Autodesk Inventor part; units mm, degrees
ref_plane "YZ Plane" through (0, 0, 0) normal (1, 0, 0) x (0, 1, 0)
ref_plane "XZ Plane" through (0, 0, 0) normal (0, 1, 0) x (-1, 0, 0)
ref_plane "XY Plane" through (0, 0, 0) normal (0, 0, 1) x (1, 0, 0)
sketch "Sketch1" plane through (0, 0, 0) normal (0, 0, 1) x (1, 0, 0)
  line L0 (457.2, 0) -> (457.2, 19.05)
  line L1 (457.2, -133.35) -> (457.2, 0)
  line L2 (0, 0) -> (0, -133.35)
  line L3 (457.2, 19.05) -> (1981.2, -133.35)
  line L4 (1789.7499, -133.35) -> (457.2, -0.095)
  line L5 (1789.7499, -133.35) -> (1981.2, -133.35)
  dimension "d3" = 19.05
  dimension "d4" = 1981.2
extrude "Extrusion1" add sketch "Sketch1" against normal blind 457.2
properties part number "Ramp1"
Geometry check sheet. Reference: the model listing, model coordinates, mm. Give positions to 0.01 mm unless a question says otherwise; leave off trailing zeros. Write each loop counter-clockwise with the first axis right and the second up, starting at its lowest first coordinate (ties: lowest second). Pieces come first, ordered by that corner, then holes.
1) Section check B-B, the plane x = 1686. Record the boundary of the cut face in (y, z) (3 decimals).
2) Section check A-A, the plane z = -96. Record the boundary of the cut face in (x, y) (3 decimals).
3) Gauge pin test, flat ends, axial feed: pin 1 (6 mm diameter, centred on x = 1481, z = -392, fed in from -Y) (3 decimals); pin 2 (2 mm diameter, centred on x = 961, z = -233, fed in from -Y) (3 decimals); pin 3 (10 mm diameter, centred on x = 1115.5, z = -358.5, fed in from -Y) (3 decimals). Record the tip position at first contact, or that the pin passes through.
4) Material ranges on L1, parallel to Y at x = 1027.5, z = -341.5 (3 decimals); L2, parallel to Y at x = 1285, z = -310 (3 decimals), recorded low to high.
Computed:
1. outline: (-122.975, -457.2) - (-103.83, -457.2) - (-103.83, 0) - (-122.975, 0) - close
2. outline: (457.2, -0.095) - (1789.75, -133.35) - (1981.2, -133.35) - (457.2, 19.05) - close
3. pin 1: stops at y = -102.775
3. pin 2: stops at y = -50.575
3. pin 3: stops at y = -66.425
4. L1: y = -57.125 to -37.98
4. L2: y = -82.875 to -63.73
